Can you work these out from the model? Positions are in its coordinate system, mm. Coordinates: 2 decimals unless noted, no trailing zeros. Order: outer loops, then holes, each group sorted by start corner. A loop starts at its lowest first (then second) coordinate and runs counter-clockwise, first axis right, second up. Notation, with made-up numbers: (31.5, 20) - (82.5, 20) arc R33 ccw to (82.5, 55) - close; hole circle Ø10 at (61.25, 32.25). An arc over 180 degrees is marked (long way). Return JSON: item names as keys, results as strings. Group by question number.
1) Imagine slicing it at A-A (x = -15.5). Write out the boundary of the cut face in (y, z), and give its area (3 significant figures).
2) Imagine slicing it at C-C (z = -91.5). Write out the boundary of the cut face in (x, y).
3) If I drill on line 1 along Y through (x, z) = (-22.25, -363.5); line 2 along Y through (x, z) = (-3.25, -144), over which ranges is the centre line in solid material (lowest first)?
```python
from build123d import *

# Parameters (mm, degrees)
EXTRUDE_1_DEPTH = 482.5


with BuildPart() as part:
    # Эскиз1 → Бобышка-Вытянуть1 (new body)
    with BuildSketch(Plane.XY):
        with BuildLine():
            Line((-27, 0), (-3, 0))
            ThreePointArc((-3, 0), (-0.878679656, -0.878679656), (0, -3))
            Line((0, -3), (0, -27))
            ThreePointArc((0, -27), (-0.878679656, -29.121320344), (-3, -30))
            Line((-3, -30), (-27, -30))
            ThreePointArc((-27, -30), (-29.121320344, -29.121320344), (-30, -27))
            Line((-30, -27), (-30, -3))
            ThreePointArc((-30, -3), (-29.121320344, -0.878679656), (-27, 0))
        make_face()
        with BuildLine():
            Line((-26, -2), (-4, -2))
            ThreePointArc((-4, -2), (-2.585786438, -2.585786438), (-2, -4))
            Line((-2, -4), (-2, -26))
            ThreePointArc((-2, -26), (-2.585786438, -27.414213562), (-4, -28))
            Line((-4, -28), (-26, -28))
            ThreePointArc((-26, -28), (-27.414213562, -27.414213562), (-28, -26))
            Line((-28, -26), (-28, -4))
            ThreePointArc((-28, -4), (-27.414213562, -2.585786438), (-26, -2))
        make_face(mode=Mode.SUBTRACT)
    extrude(amount=-EXTRUDE_1_DEPTH)


solid = part.part
```
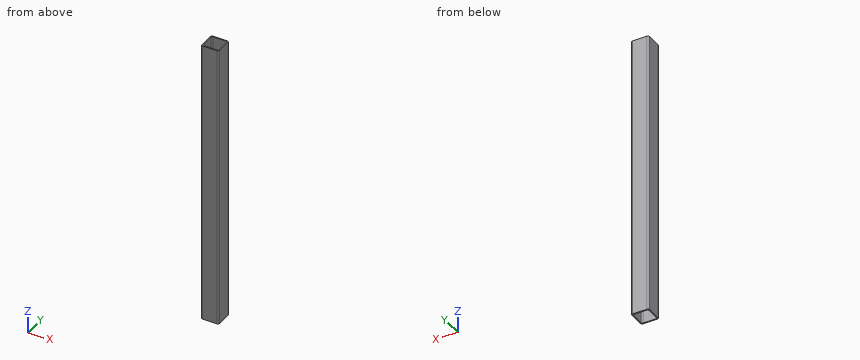
Calculated:
{
 "1": {"outline": "(-30, -482.5) - (-28, -482.5) - (-28, 0) - (-30, 0) - close; (-2, -482.5) - (0, -482.5) - (0, 0) - (-2, 0) - close", "area": "1,930 mm2"},
 "2": {"outline": "(-30, -27) arc R3 ccw to (-27, -30) - (-3, -30) arc R3 ccw to (0, -27) - (0, -3) arc R3 ccw to (-3, 0) - (-27, 0) arc R3 ccw to (-30, -3) - close; hole (-28, -26) arc R2 ccw to (-26, -28) - (-4, -28) arc R2 ccw to (-2, -26) - (-2, -4) arc R2 ccw to (-4, -2) - (-26, -2) arc R2 ccw to (-28, -4) - close"},
 "3": {"line 1": "-30 to -28, -2 to 0", "line 2": "-30 to -27.85, -2.15 to 0"}
}
